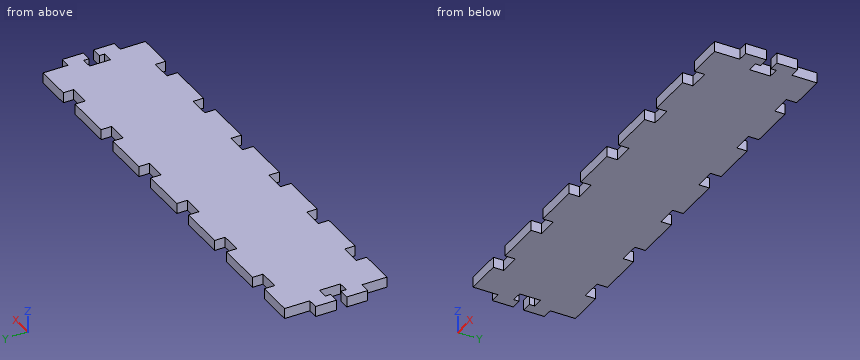
```python
from build123d import *

# Parameters (mm, degrees)
SKETCH1_W                                  = 260
SKETCH1_H                                  = 59
BOSS_EXTRUDE1_DEPTH                        = 6
SKETCH3_W                                  = 6
SKETCH3_H                                  = 6
SKETCH3_H_2                                = 14.5
CUT_EXTRUDE1_DEPTH                         = 7
SKETCH3_3_W                                = 12
SKETCH3_3_H                                = 6
CUT_EXTRUDE2_DEPTH                         = 7
MIRROR1_AT_THE_SECOND_PLANE_COPY_1_SKETC_W = 12
MIRROR1_AT_THE_SECOND_PLANE_COPY_1_SKETC_H = 6
MIRROR1_AT_THE_SECOND_PLANE_COPY_1_DEPTH   = 7


with BuildPart() as part:
    # Sketch1 → Boss-Extrude1 (new body)
    with BuildSketch(Plane.XY):
        Rectangle(SKETCH1_W, SKETCH1_H)
    extrude(amount=-BOSS_EXTRUDE1_DEPTH)

    # Sketch3 → Cut-Extrude1 (cut, through all)
    with BuildSketch(Plane.XY):
        Polygon((-124, 6), (-124, 3), (-124, -3), (-124, -6), (-118, -6), (-118, 6), align=None)
        with Locations((-127, 0)):
            Rectangle(SKETCH3_W, SKETCH3_H)
        with Locations((-127, 22.25)):
            Rectangle(SKETCH3_W, SKETCH3_H_2)
        with Locations((-127, -22.25)):
            Rectangle(SKETCH3_W, SKETCH3_H_2)
    cut_extrude1 = extrude(amount=-CUT_EXTRUDE1_DEPTH, mode=Mode.SUBTRACT)

    # Sketch3<3> → Cut-Extrude2 (cut, through all)
    with BuildSketch(Plane.XY):
        with Locations((-97.142857143, -26.5)):
            Rectangle(SKETCH3_3_W, SKETCH3_3_H)
        with Locations((-58.285714286, -26.5)):
            Rectangle(SKETCH3_3_W, SKETCH3_3_H)
        with Locations((-19.428571429, -26.5)):
            Rectangle(SKETCH3_3_W, SKETCH3_3_H)
    cut_extrude2 = extrude(amount=-CUT_EXTRUDE2_DEPTH, mode=Mode.SUBTRACT)

    # Mirror1: Cut-Extrude2 across plane
    add(cut_extrude2.mirror(Plane(origin=(0, 0, 0), x_dir=(0, 0, 1), z_dir=(1, 0, 0))), mode=Mode.SUBTRACT)

    # Mirror1 at the second plane: Cut-Extrude2 across plane
    add(cut_extrude2.mirror(Plane.ZX), mode=Mode.SUBTRACT)

    # Mirror1 at the second plane copy 1 sketc → Mirror1 at the second plane copy 1 (cut, through all)
    with BuildSketch(Plane(origin=(0, 0, 0), x_dir=(-1, 0, 0), z_dir=(0, 0, 1))):
        with Locations((-97.142857143, -26.5)):
            Rectangle(MIRROR1_AT_THE_SECOND_PLANE_COPY_1_SKETC_W, MIRROR1_AT_THE_SECOND_PLANE_COPY_1_SKETC_H)
        with Locations((-58.285714286, -26.5)):
            Rectangle(MIRROR1_AT_THE_SECOND_PLANE_COPY_1_SKETC_W, MIRROR1_AT_THE_SECOND_PLANE_COPY_1_SKETC_H)
        with Locations((-19.428571429, -26.5)):
            Rectangle(MIRROR1_AT_THE_SECOND_PLANE_COPY_1_SKETC_W, MIRROR1_AT_THE_SECOND_PLANE_COPY_1_SKETC_H)
    extrude(amount=-MIRROR1_AT_THE_SECOND_PLANE_COPY_1_DEPTH, mode=Mode.SUBTRACT)

    # Mirror2: Cut-Extrude1 across plane
    add(cut_extrude1.mirror(Plane(origin=(0, 0, 0), x_dir=(0, 0, 1), z_dir=(1, 0, 0))), mode=Mode.SUBTRACT)


solid = part.part
```
Geometry: final body of the model. Coordinates: model frame, mm. Round coordinates to 2 decimals unless told otherwise and drop trailing zeros. Order: outer loops, then holes, each group sorted by start corner. A loop starts at its lowest first (then second) coordinate and runs counter-clockwise, first axis right, second up. Notation, with made-up numbers: (10.5, -35) - (56.5, -35) arc R20 ccw to (56.5, -23) - close; hole circle Ø2 at (31.25, -40). An arc over 180 degrees is marked (long way). Use CSV: the item, a comma, the result in double quotes. Start each with the question number.
Q1. Section query B-B (y = 18.5). Return loops of the section in (x, z), and give its area (3 significant figures).
Q2. First-contact query: pin 1 (1.8 mm diameter, centred on x = -127.5, z = -2.5, fed in from +Y); pin 2 (3 mm diameter, centred on y = 26, z = -4, fed in from +X); pin 3 (3 mm diameter, centred on x = -60.5, z = -3, fed in from +Y). Flat tips, straight axial feed; report the tip coordinate or a pass-through.
Q3. Material intervals for line 1 along X through (y, z) = (5.5, -5.6); line 2 along X through (y, z) = (2, -0.85); line 3 along X through (y, z) = (16.5, -1.9), sorted ascending. Write a range as from..to.
Q4. Section query A-A (x = -95). Return loops of the section in (y, z), and give its area (3 significant figures).
Result set:
1,outline,"(-124, -6) - (124, -6) - (124, 0) - (-124, 0) - close"
1,area,"1,490 mm2"
2,pin 1,"stops at y = 15"
2,pin 2,"stops at x = 124"
2,pin 3,"stops at y = 23.5"
3,line 1,"x = -130..-124, -118..118, 124..130"
3,line 2,"x = -118..118"
3,line 3,"x = -124..124"
4,outline,"(-23.5, -6) - (23.5, -6) - (23.5, 0) - (-23.5, 0) - close"
4,area,"282 mm2"
